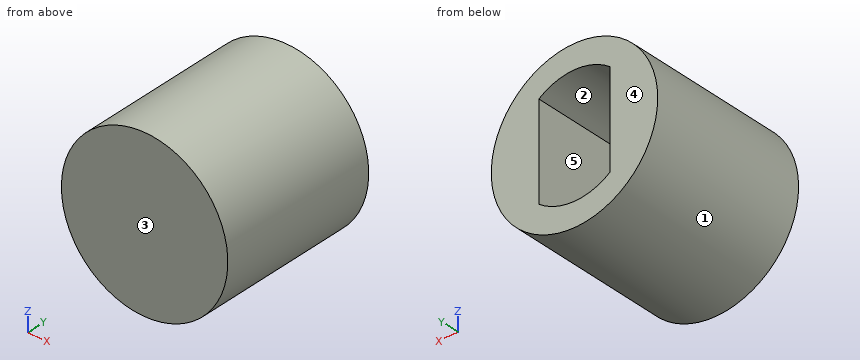
Autodesk Inventor part; units mm, degrees
ref_plane "YZ Plane" through (0, 0, 0) normal (1, 0, 0) x (0, 1, 0)
ref_plane "XZ Plane" through (0, 0, 0) normal (0, 1, 0) x (-1, 0, 0)
ref_plane "XY Plane" through (0, 0, 0) normal (0, 0, 1) x (1, 0, 0)
sketch "Sketch1" plane through (0, 0, 0) normal (0, 1, 0) x (-1, 0, 0)
  circle A0 centre (0, 0) radius 3.5
  dimension "d0" = 7
extrude "Extrusion1" add sketch "Sketch1" along normal blind 7
sketch "Sketch2" plane through (0, 7, 0) normal (0, 1, 0) x (1, 0, 0)
  circle A0 centre (0, 0) radius 2.5
  line L0 (1.5, -2.75) -> (-1.5, -2.75)
  line L1 (-1.5, -2.75) -> (-1.5, 2.75)
  line L2 (-1.5, 2.75) -> (1.5, 2.75)
  line L3 (1.5, 2.75) -> (1.5, -2.75)
  line L4 (1.5, -2.75) -> (-1.5, 2.75) construction
  line L5 (-1.5, -2.75) -> (1.5, 2.75) construction
  point P0 (1.5, -2)
  point P1 (1.5, 2)
  point P2 (-1.5, 2)
  point P3 (-1.5, -2)
  dimension "d3" = 5
  dimension "d4" = 3
  dimension "d5" = 5.5
extrude "Extrusion2" cut sketch "Sketch2" against normal blind 6 contours L3 A0 L1
properties part number "ozubeneKoleckoStepper"
Source: CAD feature listing. Evaluate the final solid. Frame: model axes, mm. Face numbers are marked on the shaded views. A direction names the side the tool comes from. Round coordinates to 2 decimals unless told otherwise and drop trailing zeros. Loops run counter-clockwise (first coordinate to the right, second up) from the corner with the lowest first, then second, coordinate; pieces in that order, holes last. Notation, with made-up numbers: M 60.5,-37.5 L 64.5,-37.5 A15 cw 64.5,-19.5 Z; hole C -37.75,15.25 d9. An arc over 180 degrees is marked long. Use a Markdown table: item, result. Add a question column.
1. Mould query, pull axis Z, two halves, no side actions, for the marked faces 1, 2 and 3. Classes: pulls with the +Z half, pulls with the -Z half, needs draft (parallel to the pull), parting line crosses it, or undercut.
2. Section query A-A on y = 1.5. Return the cut outline in (x, z).
3. Line query: line 1 (Y direction, x = -0.5, z = -1.75); line 2 (X direction, y = 6.5, z = -0.25); line 3 (Z direction, x = -0.5, y = 6.5). Output: solid intervals per line, ascending.
4. Section query B-B on z = 0. Return the cut outline in (x, y), then the cut area to 3 significant figures.
5. Section query D-D on x = -2. Return the cut outline in (y, z).
6. Section query C-C on x = 0. Return the cut outline in (y, z), then the cut area to 3 significant figures.
7. Contact query for flat-ended pins moving along their axis: P1, Ø1.5, axis at x = -2.5, y = 5.5, coming from the -Z side; P2, Ø1.5, axis at x = 0, z = 0, coming from the +Y side; P3, Ø3, axis at x = -2.5, y = 5.5, coming from the -Z side; P4, Ø3, axis at x = 2.5, z = -2.5, coming from the -Y side. Output: stop coordinate, or through.
8. Reachability of the marked faces 4 and 5 from +Z, -Z, +X, -X, +Y, -Y: full face, straight path, thin tool, end or side. Return the list, or none.
Reported:
| question | item | result |
|---|---|---|
| 1 | face 1 | parting line crosses it |
| 1 | face 2 | undercut |
| 1 | face 3 | needs draft |
| 2 | outline | C 0,0 d7; hole M -1.5,-2 A2.5 ccw 1.5,-2 L 1.5,2 A2.5 ccw -1.5,2 Z |
| 3 | line 1 | y = 0 to 1 |
| 3 | line 2 | x = -3.49 to -1.5, 1.5 to 3.49 |
| 3 | line 3 | z = -3.46 to -2.45, 2.45 to 3.46 |
| 4 | outline | M -3.5,0 L 3.5,0 L 3.5,7 L 1.5,7 L 1.5,1 L -1.5,1 L -1.5,7 L -3.5,7 Z |
| 4 | area | 31.0 mm² |
| 5 | outline | M 0,-2.87 L 7,-2.87 L 7,2.87 L 0,2.87 Z |
| 6 | outline | M 0,-3.5 L 7,-3.5 L 7,-2.5 L 1,-2.5 L 1,2.5 L 7,2.5 L 7,3.5 L 0,3.5 Z |
| 6 | area | 19.0 mm² |
| 7 | P1 | stops at z = -3.03 |
| 7 | P2 | stops at y = 1 |
| 7 | P3 | stops at z = -3.35 |
| 7 | P4 | stops at y = 0 |
| 8 | face 4 | +Z, -Z, +X, -X, +Y |
| 8 | face 5 | +Y |
